Part model, mm, in its own coordinate system. Round coordinates to 2 decimals unless told otherwise and drop trailing zeros. Write each loop counter-clockwise with the first axis right and the second up, starting at its lowest first coordinate (ties: lowest second). Pieces come first, ordered by that corner, then holes.
1) Saw through at B-B on z = 0. Write the cut outline in (x, y).
2) Drill centre lines: L1, parallel to X at y = 0.85, z = 19; L2, parallel to Z at x = 1, y = 0.1; L3, parallel to X at y = 0.4, z = 0. Where is each one in solid material? Low to high.
3) Saw through at D-D on z = -38. Write the cut outline in (x, y).
4) Pull direction X, two halves, no side cores. Call faces 1 (the flat face through (-10, 1, 10)), 2 (the cylindrical face through (0.088, 0.507, -39.998)), 3 (the cylindrical face through (34.861, 0.507, -18.566)), 4 (the cylindrical face through (-46.08, 0.49, -10.23)): +X half, -X half, draft (parallel to the pull), parting line (faces both ways), or undercut.
5) Saw through at C-C on y = 0.2. Write the cut outline in (x, z).
6) Saw through at A-A on x = 0. Write the cut outline in (y, z).
```python
from build123d import *

# Parameters (mm, degrees)
SKETCH1_R           = 47.2
BOSS_EXTRUDE1_DEPTH = 1
SKETCH2_R           = 13
CUT_EXTRUDE1_DEPTH  = 1
SKETCH4_R           = 2
CUT_EXTRUDE3_DEPTH  = 67.758370262
CIRPATTERN1_COUNT   = 6


with BuildPart() as part:
    # Sketch1 → Boss-Extrude1 (new body)
    with BuildSketch(Plane(origin=(0, 0, 0), x_dir=(1, 0, 0), z_dir=(0, 1, 0))):
        with Locations(Location((0, 0, 0), (0, 0, 270))):
            Circle(SKETCH1_R)
    extrude(amount=BOSS_EXTRUDE1_DEPTH)

    # Sketch2 → Cut-Extrude1 (cut)
    with BuildSketch(Plane(origin=(0, 1, 0), x_dir=(1, 0, 0), z_dir=(0, 1, 0))):
        with Locations(Location((0, 0, 0), (0, 0, 270))):
            Circle(SKETCH2_R)
    extrude(amount=-CUT_EXTRUDE1_DEPTH, mode=Mode.SUBTRACT)

    # Sketch4 → Cut-Extrude3 (cut, through all)
    with BuildSketch(Plane(origin=(0, 1, 0), x_dir=(1, 0, 0), z_dir=(0, 1, 0))):
        with Locations(Location((0, 38, 0), (0, 0, 270))):
            Circle(SKETCH4_R)
    cut_extrude3 = extrude(amount=-CUT_EXTRUDE3_DEPTH, mode=Mode.SUBTRACT)

    # CirPattern1: Cut-Extrude3 ×6 about axis
    cirpattern1_axis = Axis((0, 0, 0), (0, 1, 0))
    for i in range(1, CIRPATTERN1_COUNT):
        add(cut_extrude3.rotate(cirpattern1_axis, i * 360 / CIRPATTERN1_COUNT), mode=Mode.SUBTRACT)


solid = part.part
```
Completed:
1. outline: (-47.2, 0) - (-13, 0) - (-13, 1) - (-47.2, 1) - close; (13, 0) - (47.2, 0) - (47.2, 1) - (13, 1) - close
2. L1: x = -43.21 to -34.91, -30.91 to 30.91, 34.91 to 43.21
2. L2: z = -47.19 to -39.73, -36.27 to -12.96, 12.96 to 36.27, 39.73 to 47.19
2. L3: x = -47.2 to -13, 13 to 47.2
3. outline: (-28, 0) - (-2, 0) - (-2, 1) - (-28, 1) - close; (2, 0) - (28, 0) - (28, 1) - (2, 1) - close
4. face 1: draft
4. face 2: undercut
4. face 3: undercut
4. face 4: parting line
5. outline: circle Ø94.4 at (0, 0); hole circle Ø4 at (-32.91, -19); hole circle Ø4 at (-32.91, 19); hole circle Ø26 at (0, 0); hole circle Ø4 at (0, -38); hole circle Ø4 at (0, 38); hole circle Ø4 at (32.91, -19); hole circle Ø4 at (32.91, 19)
6. outline: (0, -47.2) - (1, -47.2) - (1, -40) - (0, -40) - close; (0, -36) - (1, -36) - (1, -13) - (0, -13) - close; (0, 13) - (1, 13) - (1, 36) - (0, 36) - close; (0, 40) - (1, 40) - (1, 47.2) - (0, 47.2) - close
